from build123d import *

# Parameters (mm, degrees)
SKETCH1_R           = 15
SKETCH1_R_2         = 2.5
BASE_FLANGE1_DEPTH  = 6.8
SKETCH6_R           = 3
BOSS_EXTRUDE1_DEPTH = 70


# Sheet-metal steps are written as plain solids
with BuildPart() as part:
    # Sketch1 → Base-Flange1 (new body)
    with BuildSketch(Plane.XY):
        with BuildLine():
            Line((-42.5, 0), (-5, 100))
            Line((-5, 100), (5, 100))
            Line((5, 100), (42.5, 0))
            ThreePointArc((42.5, 0), (0, -42.5), (-42.5, 0))
        make_face()
        Circle(SKETCH1_R, mode=Mode.SUBTRACT)
        with Locations((25, 0)):
            Circle(SKETCH1_R_2, mode=Mode.SUBTRACT)
        with Locations(Location((-25, 0, 0), (0, 0, 180))):
            Circle(SKETCH1_R_2, mode=Mode.SUBTRACT)
    extrude(amount=-BASE_FLANGE1_DEPTH)

    # Sketch6 → Boss-Extrude1 (add)
    with BuildSketch(Plane(origin=(0, 100, 0), x_dir=(1, 0, 0), z_dir=(0, 1, 0))):
        with Locations(Location((0, 3.4, 0), (0, 0, 270))):
            Circle(SKETCH6_R)
    extrude(amount=BOSS_EXTRUDE1_DEPTH)


solid = part.part
Model file for the job. Use its own axes, mm. A direction names the side the tool comes from. Give positions to 0.01 mm unless a question says otherwise; leave off trailing zeros. Order: outer loops, then holes, each group sorted by start corner. A loop starts at its lowest first (then second) coordinate and runs counter-clockwise, first axis right, second up. Notation, with made-up numbers: (-7, 81.5) - (4, 81.5) arc R13 ccw to (4, 101.5) - close; hole circle Ø3 at (-3, -31). An arc over 180 degrees is marked (long way). Write item = value, one per line. Start each with the question number.
1. Cut at D-D, the plane y = 84. List the corners of the cut face in (x, z).
2. Which spindle directions (+Z, -Z, +X, -X, +Y, -Y) get a long thin tool onto all of the face, cutting with end or side? Do faces 5 (the flat face through (-2.3, 100, -1.1)), 6 (the cylindrical face through (22.5, 0.1, -3.4)). Say none if no direction does.
3. Cut at C-C, the plane x = -9. List the corners of the cut face in (y, z).
4. Probe line 1 along Y through (x, z) = (0, -4.5); line 2 along X through (y, z) = (154, -3.5); line 3 along X through (y, z) = (2, -5.25). List the from-to ranges inside material, lowest first.
5. Two-plate mould, pull along Y, no slides. Class faces 1 (the cylindrical face through (-14.985, 0.66, -3.352)), 2 (the cylindrical face through (0.93, -42.49, -3.35)), 3 (the flat face through (-24.012, 49.3, -3.352)), 4 (the flat face through (-9, 14, -6.8)): pulls with the +Y half, pulls with the -Y half, needs draft (parallel to the pull), parting line crosses it, or undercut.
6. Drop flat-ended pins along their axis: P1, Ø1.5, axis at x = -19, z = -3.5, coming from the -Y side; P2, Ø1, axis at x = 19, z = -1, coming from the -Y side; P3, Ø1.5, axis at y = 139.5, z = -2.5, coming from the +X side. Give the stop position or say it passes through.
7. Cut at A-A, the plane z = -3.4. List the corners of the cut face in (x, y), and give its area (3 significant figures).
8. Cut at B-B, the plane y = 11. List the corners of the cut face in (x, z) (3 decimals).
Taken from the geometry:
q1.outline = (-11, -6.8) - (11, -6.8) - (11, 0) - (-11, 0) - close
q2.face_5 = +Y
q2.face_6 = +Z, -Z
q3.outline = (-41.54, -6.8) - (-12, -6.8) - (-12, 0) - (-41.54, 0) - close; (12, -6.8) - (89.33, -6.8) - (89.33, 0) - (12, 0) - close
q4.line_1 = -42.5 to -15, 15 to 170
q4.line_2 = -3 to 3
q4.line_3 = -41.75 to -26.5, -23.5 to -14.87, 14.87 to 23.5, 26.5 to 41.75
q5.face_1 = undercut
q5.face_2 = pulls with the -Y half
q5.face_3 = pulls with the +Y half
q5.face_4 = needs draft
q6.P1 = -38.38
q6.P2 = -38.26
q6.P3 = 3
q7.outline = (-42.5, 0) arc R42.5 ccw to (42.5, 0) - (5, 100) - (3, 100) - (3, 170) - (-3, 170) - (-3, 100) - (-5, 100) - close; hole circle Ø5 at (-25, 0); hole circle Ø30 at (0, 0); hole circle Ø5 at (25, 0)
q7.area = 7,260 mm²
q8.outline = (-38.375, -6.8) - (-10.198, -6.8) - (-10.198, 0) - (-38.375, 0) - close; (10.198, -6.8) - (38.375, -6.8) - (38.375, 0) - (10.198, 0) - close
